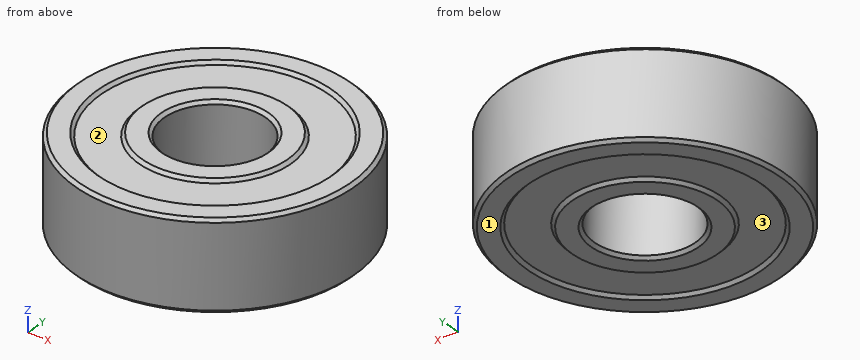
```python
from build123d import *

# Parameters (mm, degrees)
CHAMFER_SIZE = 0.25


with BuildPart() as part:
    # Sketch → Revolution (revolve)
    with BuildSketch(Plane.XZ):
        Polygon((4, -3.5), (5.75, -3.5), (6, -3.25), (9, -3.25), (9.25, -3.5), (11, -3.5), (11, 3.5), (9.25, 3.5), (9, 3.25), (6, 3.25), (5.75, 3.5), (4, 3.5), align=None)
    revolve(axis=Axis((0, 0, 0), (0, 0, 1)))

    # Chamfer
    chamfer_edges = [part.edges().sort_by_distance(p)[0] for p in [
        (-4, 0, -3.5),
        (-4, 0, 3.5),
        (-11, 0, -3.5),
        (-11, 0, 3.5),
    ]]
    chamfer(chamfer_edges, length=CHAMFER_SIZE)


solid = part.part
```
Design review of the part built by this model. Coordinates are the model's own, in mm. Face numbers are marked on the shaded views. A direction names the side the tool comes from. Coordinates: 2 decimals unless noted, no trailing zeros. Write each loop counter-clockwise with the first axis right and the second up, starting at its lowest first coordinate (ties: lowest second). Pieces come first, ordered by that corner, then holes. Notation, with made-up numbers: M 3,-7 L 36,-7 A29 ccw 36,14 Z; hole C 22,-21.5 d6. An arc over 180 degrees is marked long. Answer as a JSON object with one key per item and string values.
Item 1: Wall thickness on probe 1 along Y at (x, z) = (0, -1.25); probe 2 along Z at (x, y) = (3.5, -7.75); probe 3 along X at (y, z) = (-1.75, -3): over which ranges is each line inside the solid? List them lowest first.
Outcome:
{"probe 1": "-11 to -4, 4 to 11", "probe 2": "-3.25 to 3.25", "probe 3": "-10.86 to -3.6, 3.6 to 10.86"}
Item 2: Machinability: for the marked faces 1, 2 and 3, which of the approach directions +Z, -Z, +X, -X, +Y, -Y give a long, thin tool a straight path to every point of the face, cutting with its end or side? Answer none if there is none.
Outcome:
{"face 1": "-Z, +X, -X, +Y, -Y", "face 2": "+Z", "face 3": "-Z"}
Item 3: Add section C-C, the plane z = -2.5. Give the boundary of the cut face in (x, y).
Outcome:
{"outline": "C 0,0 d22; hole C 0,0 d8"}
Item 4: Insertion check: pin 1 Ø2 at (y, z) = (8.5, 1.5) entering from +X; pin 2 Ø1 at (x, z) = (5, -2.5) entering from -Y; pin 3 Ø3 at (y, z) = (2.5, 1) entering from +X. Each pin has a flat end and moves straight along its axis. Give the tip position at first contact, or say it passes through.
Outcome:
{"pin 1": "x = 8.05", "pin 2": "y = -10.04", "pin 3": "x = 10.95"}
